Study the drawing (mm; zero at the part's minimum x, y, z) and answer. A direction names the side the tool comes from. Round coordinates to 2 decimals unless told otherwise and drop trailing zeros. Write each loop counter-clockwise with the first axis right and the second up, starting at its lowest first coordinate (ties: lowest second). Pieces come first, ordered by that corner, then holes. Notation, with made-up numbers: M -14,-5 L 7,-5 A17 ccw 7,8 Z; hole C 87,-35 d11. An arc over 180 degrees is marked long. Write each question's results on one line, items separated by ' | '.
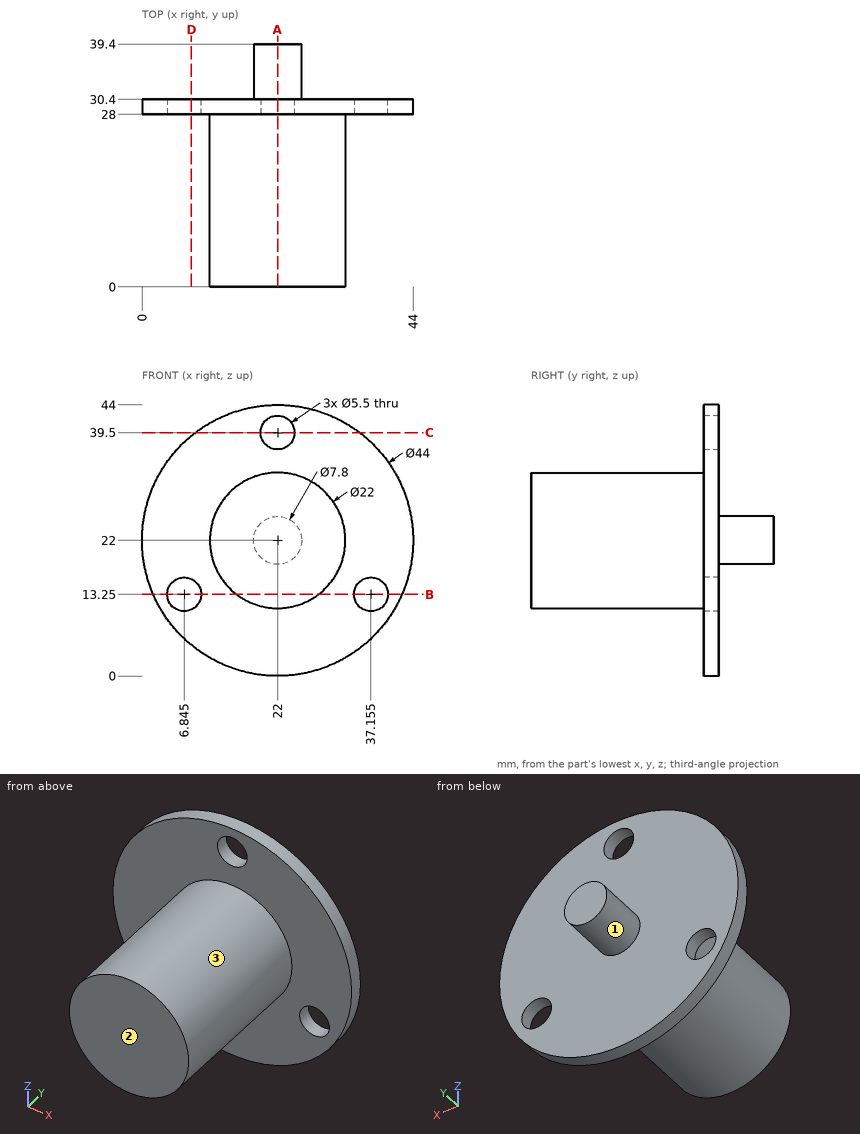
1) Section D-D (x = 8) is taken. Determine the outline of the cut face in (y, z) (1 decimal).
Return value:
outline: M 28,5 L 30.4,5 L 30.4,10.8 L 28,10.8 Z; M 28,15.7 L 30.4,15.7 L 30.4,39 L 28,39 Z
2) Each of these flat-tipped pins is pushed along its axis until it touches: pin 1 (2 mm diameter, centred on x = 5.5, z = 21.5, fed in from +Y); pin 2 (7 mm diameter, centred on x = 37.16, z = 13.25, fed in from -Y); pin 3 (8 mm diameter, centred on x = 32.5, y = 6, fed in from -Z) (1 decimal); pin 4 (4.5 mm diameter, centred on x = 22, z = 39.5, fed in from +Y). Where does it stop, or does it pass through?
Return value:
pin 1: y = 30.4 | pin 2: y = 28 | pin 3: z = 13.1 | pin 4: through
3) Section B-B (z = 13.25) is taken. Determine the outline of the cut face in (x, y) (1 decimal).
Return value:
outline: M 1.8,28 L 4.1,28 L 4.1,30.4 L 1.8,30.4 Z; M 9.6,28 L 15.3,28 L 15.3,0 L 28.7,0 L 28.7,28 L 34.4,28 L 34.4,30.4 L 9.6,30.4 Z; M 39.9,28 L 42.2,28 L 42.2,30.4 L 39.9,30.4 Z
4) Section A-A (x = 22) is taken. Determine the outline of the cut face in (y, z).
Return value:
outline: M 0,11 L 28,11 L 28,0 L 30.4,0 L 30.4,18.1 L 39.4,18.1 L 39.4,25.9 L 30.4,25.9 L 30.4,36.75 L 28,36.75 L 28,33 L 0,33 Z; M 28,42.25 L 30.4,42.25 L 30.4,44 L 28,44 Z
5) Find the intervals of material crossed by line 1 (X direction, y = 28.6, z = 13.25) (1 decimal); line 2 (Y direction, x = 28, z = 6.5); line 3 (Z direction, x = 22, y = 29), in increasing order.
Return value:
line 1: 1.8 to 4.1, 9.6 to 34.4, 39.9 to 42.2 | line 2: 28 to 30.4 | line 3: 0 to 36.75, 42.25 to 44
6) Section C-C (z = 39.5) is taken. Determine the outline of the cut face in (x, y).
Return value:
outline: M 8.67,28 L 19.25,28 L 19.25,30.4 L 8.67,30.4 Z; M 24.75,28 L 35.33,28 L 35.33,30.4 L 24.75,30.4 Z
7) A tool of negligible diameter and unlimited length cuts with its end or side. For the marked faces 1, 2 and 3, from which of +Z, -Z, +X, -X, +Y, -Y can it reach the whole face along a straight path? Write none if from no direction.
Return value:
face 1: +Y | face 2: +Z, -Z, +X, -X, -Y | face 3: -Y
